Geometry check sheet. Reference: the model listing, model coordinates, mm. A direction names the side the tool comes from. Give positions to 0.01 mm unless a question says otherwise; leave off trailing zeros. Loops run counter-clockwise (first coordinate to the right, second up) from the corner with the lowest first, then second, coordinate; pieces in that order, holes last. Notation, with made-up numbers: (81.25, -20) -> (130.25, -20) arc R17 ccw to (130.25, -1) -> close; hole circle Ø6 at (-27, -28.75). An arc over 180 degrees is marked (long way). Write each question's results on one line, items separated by ' | '. Start each with the question number.
1) Draft check along Z on faces 3 (the face through (285.154, 103.95, -362.811)), 4 (the face through (191, 15, 12.605)), 5 (the face through (-6.02, 15, -190)). Enter one of: pulls with the +Z half, pulls with the -Z half, needs draft (parallel to the pull), parting line crosses it, or undercut.
2) Sectioned sample at D-D on z = -113. Record the cut outline in (x, y), then the cut area to 3 significant figures.
3) Scan lines: line 1 (Z direction, x = 55, y = 55.5); line 2 (Y direction, x = 161, z = -58.5); line 3 (X direction, y = 103.5, z = -356). Record each from-to range of solid material in increasing order. Write a range as from..to.
4) Sectioned sample at C-C on y = 42. Record the cut outline in (x, z).
5) Sectioned sample at A-A on z = -17.5. Record the cut outline in (x, y).
6) Depth check by flat-ended pin: pin 1 (2 mm diameter, centred on x = 200, z = -321.5, fed in from +Y). Enter the tip coordinate at first touch or a pass-through.
7) Set-up check for faces 1 (the face through (32.822, 103.95, -47.396)), 2 (the face through (305, 180, -33)): record each of +Z, -Z, +X, -X, +Y, -Y from which the full face is reachable in a straight line by a thin tool's end or side.
8) Sectioned sample at B-B on x = 314.5. Record the cut outline in (y, z).
Autodesk Inventor part; units mm, degrees
ref_plane "YZ Plane" through (0, 0, 0) normal (1, 0, 0) x (0, 1, 0)
ref_plane "XZ Plane" through (0, 0, 0) normal (0, 1, 0) x (-1, 0, 0)
ref_plane "XY Plane" through (0, 0, 0) normal (0, 0, 1) x (1, 0, 0)
sketch "Sketch1" plane through (0, 0, 0) normal (0, 1, 0) x (-1, 0, 0)
  line L0 (6.0199, 12.6049) -> (-393.9801, 12.6049)
  line L1 (-393.9801, 12.6049) -> (-393.9801, -387.3951)
  line L2 (-393.9801, -387.3951) -> (6.0199, -387.3951)
  line L3 (6.0199, -387.3951) -> (6.0199, 12.6049)
  point P0 (0, 0)
  dimension "d0" = 400
  dimension "d1" = 400
  dimension "d2" = 400
extrude "Extrusion1" add sketch "Sketch1" along normal blind 30
sketch "Sketch2" plane through (0, 30, 0) normal (0, 1, 0) x (1, 0, 0)
  circle A0 centre (52.6612, 32.1839) radius 25
  circle A1 centre (304.9932, 32.1839) radius 25
  circle A2 centre (304.9932, 347.5989) radius 25
  circle A3 centre (52.6612, 354.7675) radius 25
  point P0 (0, 0)
  dimension "d5" = 50
  dimension "d6" = 50
  dimension "d7" = 50
  dimension "d8" = 50
extrude "Extrusion2" add sketch "Sketch2" along normal blind 150
sketch "Sketch3" plane through (0, 0, 0) normal (0, -1, 0) x (1, 0, 0)
  point P0 (0, 0)
sketch "Sketch4" plane through (0, 30, 0) normal (0, 1, 0) x (1, 0, 0)
  point P0 (0, 0)
  point P1 (172.4185, 228.0493)
hole "Hole1" at (172.4185, 30, -228.0493) direction (0, -1, 0) diameter 17.894 depth 53.975 tip angle 118
properties part number "base1"
Result:
1) face 3: undercut | face 4: pulls with the +Z half | face 5: needs draft
2) outline: (-6.02, 0) -> (393.98, 0) -> (393.98, 30) -> (-6.02, 30) -> close | area: 12,000 mm^2
3) line 1: -379.66..-329.88, -57.07..-7.29 | line 2: 0..30 | line 3: 27.69..77.63, 281.45..328.54
4) outline: circle Ø50 at (52.66, -354.77); circle Ø50 at (52.66, -32.18); circle Ø50 at (304.99, -347.6); circle Ø50 at (304.99, -32.18)
5) outline: (-6.02, 0) -> (393.98, 0) -> (393.98, 30) -> (325.23, 30) -> (325.23, 180) -> (284.76, 180) -> (284.76, 30) -> (72.89, 30) -> (72.89, 180) -> (32.43, 180) -> (32.43, 30) -> (-6.02, 30) -> close
6) pin 1: y = 30
7) face 1: +Y | face 2: +Z, -Z, +X, -X, +Y
8) outline: (0, -387.4) -> (30, -387.4) -> (30, -370.72) -> (180, -370.72) -> (180, -324.48) -> (30, -324.48) -> (30, -55.31) -> (180, -55.31) -> (180, -9.06) -> (30, -9.06) -> (30, 12.6) -> (0, 12.6) -> close
